CAD build for the part. Positions are in the model's coordinates, mm. A direction names the side the tool comes from. Round coordinates to 2 decimals unless told otherwise and drop trailing zeros. Loops run counter-clockwise (first coordinate to the right, second up) from the corner with the lowest first, then second, coordinate; pieces in that order, holes last. Notation, with made-up numbers: M 87,-28 L 92,-28 A34 ccw 92,10 Z; hole C 25,36.25 d4. An arc over 180 degrees is marked long. Use a Markdown table: item, result. Add a question column.
(1) Which spindle directions (+Z, -Z, +X, -X, +Y, -Y) get a long thin tool onto all of the face, cutting with end or side? Do faces 5 (the face through (-17, -33, 0)), 6 (the face through (-35, -3, 15)), 7 (the face through (-3, 35, 15)). Say none if no direction does.
(2) Two-plate mould, pull along Y, no slides. Class faces 1 (the face through (0, 0, 0)), 2 (the face through (-26, -26, 15)), 3 (the face through (-35, 0, 10)), 4 (the face through (42.016, -13.231, -2.465)): released by +Y, released by -Y, zero draft, split by the parting line, or undercut.
(3) Flat gauge pins, fed straight in: P1, Ø2, axis at x = -30, z = 15.5, coming from the +Y side; P2, Ø4, axis at x = -3.5, y = -17.5, coming from the +Z side; P3, Ø2.5, axis at x = -35, y = -1.5, coming from the +Z side. Where does each tip first touch, or does it go through?
(4) Band-saw the part on A-A, the plane y = 0. Write the cut outline in (x, z).
(5) Wall check: L1, parallel to Y at x = 0, z = 7.75; L2, parallel to Y at x = 9, z = 9.5. Give the ranges that are in metal, low to high.
(6) Band-saw the part on C-C, the plane z = 6.75. Write the cut outline in (x, y).
from build123d import *

# Parameters (mm, degrees)
F0_R      = 36.5
F0_R_2    = 33.5
F1_DEPTH  = 20
F2_R      = 36.5
F3_DEPTH  = 5
F3_TAPER  = -25
F4_R      = 33.5
F5_DEPTH  = 25
F6_R      = 44.05
F7_DEPTH  = 5
F10_DEPTH = 25


with BuildPart() as f1:
    # F0 (on Top) → F1 (new body)
    with BuildSketch(Plane.XY):
        Circle(F0_R)
        Circle(F0_R_2, mode=Mode.SUBTRACT)
    extrude(amount=F1_DEPTH)

    # F2 (on face) → F3 (join)
    with BuildSketch(Plane.XY.offset(20)):
        Circle(F2_R)
    extrude(amount=-F3_DEPTH, taper=F3_TAPER)

    # F4 (on face) → F5 (cut)
    with BuildSketch(Plane(origin=(0, 0, 15), x_dir=(1, 0, 0), z_dir=(0, 0, -1))):
        Circle(F4_R)
    extrude(amount=-F5_DEPTH, mode=Mode.SUBTRACT)

    # F6 (on face) → F7 (join)
    with BuildSketch(Plane(origin=(0, 0, 0), x_dir=(1, 0, 0), z_dir=(0, 0, -1))):
        Circle(F6_R)
    extrude(amount=F7_DEPTH)

    # F9 (on mid) → F10 (cut)
    with BuildSketch(Plane.XY.offset(10)):
        with BuildLine():
            Line((35.05, 3), (3, 3))
            Line((3, 3), (3, 35.05))
            Line((3, 35.05), (3, 38.3829389182))
            ThreePointArc((3, 38.3829389182), (0, 38.5), (-3, 38.3829389182))
            Line((-3, 38.3829389182), (-3, 35.05))
            Line((-3, 35.05), (-3, 3))
            Line((-3, 3), (-38.3829389182, 3))
            Line((-38.3829389182, 3), (-61.3953992724, 3))
            Line((-61.3953992724, 3), (-61.3953992724, -3))
            Line((-61.3953992724, -3), (-3, -3))
            Line((-3, -3), (-3, -40.2699470416))
            Line((-3, -40.2699470416), (-3, -53.7798181176))
            Line((-3, -53.7798181176), (3, -53.7798181176))
            Line((3, -53.7798181176), (3, -40.2699470416))
            Line((3, -40.2699470416), (3, -29.05))
            Line((3, -29.05), (3, -3))
            Line((3, -3), (61.3953992724, -3))
            Line((61.3953992724, -3), (61.3953992724, 3))
            Line((61.3953992724, 3), (38.3829389182, 3))
            Line((38.3829389182, 3), (35.05, 3))
        make_face()
        with BuildLine():
            ThreePointArc((-3, 38.3829389182), (0, 38.5), (3, 38.3829389182))
            Line((3, 38.3829389182), (3, 40.2699470416))
            Line((3, 40.2699470416), (3, 53.7798181176))
            Line((3, 53.7798181176), (-3, 53.7798181176))
            Line((-3, 53.7798181176), (-3, 40.2699470416))
            Line((-3, 40.2699470416), (-3, 38.3829389182))
        make_face()
    extrude(amount=F10_DEPTH, mode=Mode.SUBTRACT)


solid = f1.part
Return value:
| question | item | result |
|---|---|---|
| 1 | face 5 | none |
| 1 | face 6 | +Z, +X, -X |
| 1 | face 7 | +Z, +Y, -Y |
| 2 | face 1 | undercut |
| 2 | face 2 | zero draft |
| 2 | face 3 | undercut |
| 2 | face 4 | split by the parting line |
| 3 | P1 | y = 25.67 |
| 3 | P2 | z = 0 |
| 3 | P3 | z = 10 |
| 4 | outline | M -44.05,-5 L 44.05,-5 L 44.05,0 L 36.5,0 L 36.5,10 L 33.5,10 L 33.5,0 L -33.5,0 L -33.5,10 L -36.5,10 L -36.5,0 L -44.05,0 Z |
| 5 | L1 | -36.5 to -33.5, 33.5 to 36.5 |
| 5 | L2 | -35.37 to -32.27, 32.27 to 35.37 |
| 6 | outline | C 0,0 d73; hole C 0,0 d67 |
